Check sheet for the modelled part. Datum: model origin and axes. Units: mm. A direction names the side the tool comes from. Give positions to 0.01 mm unless a question says otherwise; leave off trailing zeros. Loops run counter-clockwise (first coordinate to the right, second up) from the corner with the lowest first, then second, coordinate; pieces in that order, holes last. Notation, with made-up numbers: (51, 81.25) -> (58, 81.25) arc R22 ccw to (58, 102.25) -> close; hole circle Ø5 at (50, 75). An arc over 180 degrees is marked (long way). Write each question's results on one line, items separated by ' | '. Start each with the question number.
1. Material ranges on L1, parallel to X at y = 13, z = 12; L2, parallel to X at y = -13.5, z = 17; L3, parallel to Z at x = 3, y = 15.5, recorded low to high. Write a range as from..to.
2. Tool access check on faces 1 (the face through (122.56, 11.06, -11.56)), 2 (the face through (111.468, -12.165, -13.267)), 3 (the face through (122.56, 1.553, 21.075)). Record the directions out of +Z, -Z, +X, -X, +Y, -Y that give a thin tool (end or side, any length) a straight path to the whole face; none if there is none.
3. Mould release check, pull along Y, two halves, no side actions. Record for faces 4 (the face through (122.56, -21.35, -1.28)), 5 (the face through (4.19, -13.976, 14.868)), 6 (the face through (4, 0, -21)): +Y half, -Y half, draft (parallel to the pull), parting line (faces both ways), or undercut.
4. Cross-section at B-B on x = 68. Record the boundary of the cut face in (y, z).
5. Gauge pin test, flat ends, axial feed: pin 1 Ø6 at (x, z) = (61, -10.5) entering from -Y; pin 2 Ø5.5 at (y, z) = (15.5, -15.5) entering from -X; pin 3 Ø12 at (x, y) = (102, 1.5) entering from -Z. Record the tip position at first contact, or that the pin passes through.
from build123d import *

# Parameters (mm, degrees)
SKETCH_1_W                 = 42
SKETCH_1_H                 = 42
EXTRUDE_1_DEPTH            = 8.5
SKETCH_2_R                 = 47.208301361
CUT_EXTRUDE_1_DEPTH        = 8.5
SKETCH_3_R                 = 11
EXTRUDE_2_DEPTH            = 2
SKETCH_4_R                 = 4
EXTRUDE_3_DEPTH            = 16.8
CUT_EXTRUDE_START          = -15
CUT_EXTRUDE_2_DEPTH        = 15
SKETCH_7_R                 = 18
EXTRUDE_4_DEPTH            = 101.2
SKETCH_8_R                 = 16.5
EXTRUDE_5_DEPTH            = 0.5
EXTRUDE_START              = 2.5
SKETCH_9_R                 = 18
EXTRUDE_6_DEPTH            = 2.5
EXTRUDE_7_DEPTH            = 20
HOLE_WIZARD_M4_1_D         = 3.3
PATTERN_LINEAR_1_OUTLINE_R = 1.65
PATTERN_LINEAR_1_DEPTH     = 8.5
SKETCH_13_W                = 1
SKETCH_13_H                = 1


# Read off the part's stored shape, not the designer's step: 阵列(线性)1
with BuildPart() as part:
    # 草图1 → 凸台-拉伸1 (new body)
    with BuildSketch(Plane(origin=(0, 0, 0), x_dir=(0, 0, -1), z_dir=(1, 0, 0))):
        Rectangle(SKETCH_1_W, SKETCH_1_H)
    extrude(amount=EXTRUDE_1_DEPTH)

    # 草图2 → 切除-拉伸1 (cut)
    with BuildSketch(Plane.ZY):
        Circle(SKETCH_2_R)
        Polygon((39.597979746, 0), (0, 39.597979746), (-39.597979746, 0), (0, -39.597979746), align=None, mode=Mode.SUBTRACT)
    extrude(amount=-CUT_EXTRUDE_1_DEPTH, mode=Mode.SUBTRACT)

    # 草图3 → 凸台-拉伸2 (add)
    with BuildSketch(Plane.ZY):
        Circle(SKETCH_3_R)
    extrude(amount=EXTRUDE_2_DEPTH)

    # 草图4 → 凸台-拉伸3 (add)
    with BuildSketch(Plane.ZY.offset(2)):
        Circle(SKETCH_4_R)
    extrude(amount=EXTRUDE_3_DEPTH)

    # 草图5 → 切除-拉伸2 (cut)
    with BuildSketch(Plane.ZY.offset(18.8).offset(CUT_EXTRUDE_START)):
        with BuildLine():
            Line((-2.645751311, 3), (2.645751311, 3))
            ThreePointArc((2.645751311, 3), (0, 4), (-2.645751311, 3))
        make_face()
    extrude(amount=CUT_EXTRUDE_2_DEPTH, mode=Mode.SUBTRACT)

    # 草图7 → 凸台-拉伸4 (add)
    with BuildSketch(Plane.ZY.offset(-109.7)):
        Circle(SKETCH_7_R)
    extrude(amount=EXTRUDE_4_DEPTH)

    # 草图8 → 凸台-拉伸5 (add)
    with BuildSketch(Plane(origin=(109.7, 0, 0), x_dir=(0, 0, -1), z_dir=(1, 0, 0))):
        Circle(SKETCH_8_R)
    extrude(amount=EXTRUDE_5_DEPTH)

    # 草图9 → 凸台-拉伸6 (add)
    with BuildSketch(Plane(origin=(110.2, 0, 0), x_dir=(0, 0, -1), z_dir=(1, 0, 0)).offset(EXTRUDE_START)):
        with Locations(Location((0, 0, 0), (0, 0, 180))):
            Circle(SKETCH_9_R)
    extrude(amount=-EXTRUDE_6_DEPTH)

    # 草图10 → 凸台-拉伸7 (add)
    with BuildSketch(Plane(origin=(112.7, 0, 0), x_dir=(0, 0, -1), z_dir=(1, 0, 0))):
        with BuildLine():
            Line((-11.313708499, 11.313708499), (-31.112698372, -8.485281374))
            Line((-31.112698372, -8.485281374), (-8.485281374, -31.112698372))
            Line((-8.485281374, -31.112698372), (11.313708499, -11.313708499))
            ThreePointArc((11.313708499, -11.313708499), (11.313708499, 11.313708499), (-11.313708499, 11.313708499))
        make_face()
    extrude(amount=EXTRUDE_7_DEPTH)

    # M4 螺纹孔1 (through all)
    with Locations(Plane(origin=(0, 15.5, -15.5), x_dir=(0, 0, -1), z_dir=(-1, 0, 0))):
        with Locations((0, 0)):
            Hole(HOLE_WIZARD_M4_1_D / 2)

    # 阵列(线性)1 outline → 阵列(线性)1 (cut)
    with BuildSketch(Plane.YZ):
        with Locations((-15.5, -15.5)):
            Circle(PATTERN_LINEAR_1_OUTLINE_R)
        with Locations((15.5, 15.5)):
            Circle(PATTERN_LINEAR_1_OUTLINE_R)
        with Locations((-15.5, 15.5)):
            Circle(PATTERN_LINEAR_1_OUTLINE_R)
    extrude(amount=PATTERN_LINEAR_1_DEPTH, mode=Mode.SUBTRACT)

    # 草图13 → 切除-旋转1 (revolve, cut)
    with BuildSketch(Plane(origin=(0, 0, 0), x_dir=(1, 0, 0), z_dir=(0, 1, 0)), mode=Mode.PRIVATE) as cut_revolve_1_sk:
        with Locations((47.2, 17.5)):
            Rectangle(SKETCH_13_W, SKETCH_13_H)
    revolve(cut_revolve_1_sk.sketch.rotate(Axis((8.5, 0, 0), (1, 0, 0)), 180), axis=Axis((8.5, 0, 0), (1, 0, 0)), mode=Mode.SUBTRACT)


solid = part.part
Geometry says:
1) L1: 0..46.7, 47.7..109.7, 110.2..112.7 | L2: 0..8.5, 112.7..132.7 | L3: -21..-17.15, -13.85..13.85, 17.15..21
2) face 1: +X | face 2: none | face 3: +Z, +X, +Y
3) face 4: -Y half | face 5: undercut | face 6: draft
4) outline: circle Ø36 at (0, 0)
5) pin 1: y = -16.36 | pin 2: x = 0 | pin 3: z = -18
